Read the model definition and answer for the solid it produces. Units are mm, in the model's axes. Give positions to 0.01 mm unless a question says otherwise; leave off trailing zeros. Write each loop counter-clockwise with the first axis right and the second up, starting at its lowest first coordinate (ties: lowest second). Pieces come first, ordered by that corner, then holes. Notation, with made-up numbers: (-16, 17.25) - (-7, 17.25) arc R13 cw to (-7, 34.25) - close; hole circle Ø7 at (66, -26.75). An arc over 180 degrees is marked (long way). Answer as CSV lines item,"result".
```python
from build123d import *

# Parameters (mm, degrees)
F0_R      = 25.320305
F1_DEPTH  = 77.978
F1_FACE_R = 25.320305
F2_DEPTH  = 75.946


with BuildPart() as f1:
    # F0 (on Front) → F1 (new body)
    with BuildSketch(Plane.XZ):
        with BuildLine():
            Line((-39.191756, 46.791889), (-39.191756, -46.791889))
            Line((-39.191756, -46.791889), (39.191756, -46.791889))
            Line((39.191756, -46.791889), (39.191756, 46.791889))
            ThreePointArc((39.191756, 46.791889), (0, 85.983645), (-39.191756, 46.791889))
        make_face()
        with Locations((0, 46.791889)):
            Circle(F0_R, mode=Mode.SUBTRACT)
    extrude(amount=-F1_DEPTH)

    # F1_face (on face) → F2 (join)
    with BuildSketch(Plane(origin=(0, 0, 7.600639), x_dir=(1, 0, 0), z_dir=(0, -1, 0))):
        with BuildLine():
            Line((-39.191756, 39.19125), (-39.191756, -54.392528))
            Line((-39.191756, -54.392528), (39.191756, -54.392528))
            Line((39.191756, -54.392528), (39.191756, 39.19125))
            ThreePointArc((39.191756, 39.19125), (0, 78.383006), (-39.191756, 39.19125))
        make_face()
        with Locations((0, 39.19125)):
            Circle(F1_FACE_R, mode=Mode.SUBTRACT)
    extrude(amount=F2_DEPTH)


solid = f1.part
```
(1) A cutting plane is placed at B-B (y = -36). Write down the section's boundary in (x, z).
Worked out:
outline,"(-39.19, -46.79) - (39.19, -46.79) - (39.19, 46.79) arc R39.19 ccw to (-39.19, 46.79) - close; hole circle Ø50.64 at (0, 46.79)"
(2) A cutting plane is placed at C-C (z = 36.5). Write down the section's boundary in (x, y).
Worked out:
outline,"(-39.19, -75.95) - (-23.13, -75.95) - (-23.13, 77.98) - (-39.19, 77.98) - close; (23.13, -75.95) - (39.19, -75.95) - (39.19, 77.98) - (23.13, 77.98) - close"
(3) A cutting plane is placed at A-A (x = 0). Write down the section's boundary in (y, z), and give its area (3 significant figures).
Worked out:
outline,"(-75.95, -46.79) - (77.98, -46.79) - (77.98, 21.47) - (-75.95, 21.47) - close; (-75.95, 72.11) - (77.98, 72.11) - (77.98, 85.98) - (-75.95, 85.98) - close"
area,"12,600 mm^2"
(4) A cutting plane is placed at D-D (z = 76). Write down the section's boundary in (x, y), and give its area (3 significant figures).
Worked out:
outline,"(-26.13, -75.95) - (26.13, -75.95) - (26.13, 77.98) - (-26.13, 77.98) - close"
area,"8,040 mm^2"
(5) The mould has two halves that part along X. Classify faces 1 (the flat face through (-39.192, 2, 1)), 2 (the flat face through (-1, 2, -46.792)), 3 (the cylindrical face through (-3.296, 2.093, 71.897)): +X half, -X half, draft (parallel to the pull), parting line (faces both ways), or undercut.
Worked out:
face 1,"-X half"
face 2,"draft"
face 3,"undercut"
(6) Find the intervals of material crossed by L1, parallel to Z at x = 0, y = 44.5; L2, parallel to X at y = 35, z = 57; L3, parallel to Z at x = 17, y = -48, in increasing order.
Worked out:
L1,"z = -46.79 to 21.47, 72.11 to 85.98"
L2,"x = -37.84 to -23.17, 23.17 to 37.84"
L3,"z = -46.79 to 28.03, 65.56 to 82.1"
(7) Each of these flat-tipped pins is pushed along its axis until it touches: P1, Ø6, axis at x = 18, y = -16, coming from the +Z side; P2, Ø1, axis at x = 26.5, y = -17.5, coming from the +Z side; P3, Ø10, axis at x = -18, y = -57, coming from the +Z side; P4, Ø6, axis at x = -22, z = 38.5, coming from the -Y side. Where does it stop, or does it pass through?
Worked out:
P1,"stops at z = 83"
P2,"stops at z = 76.12"
P3,"stops at z = 83.76"
P4,"stops at y = -75.95"
